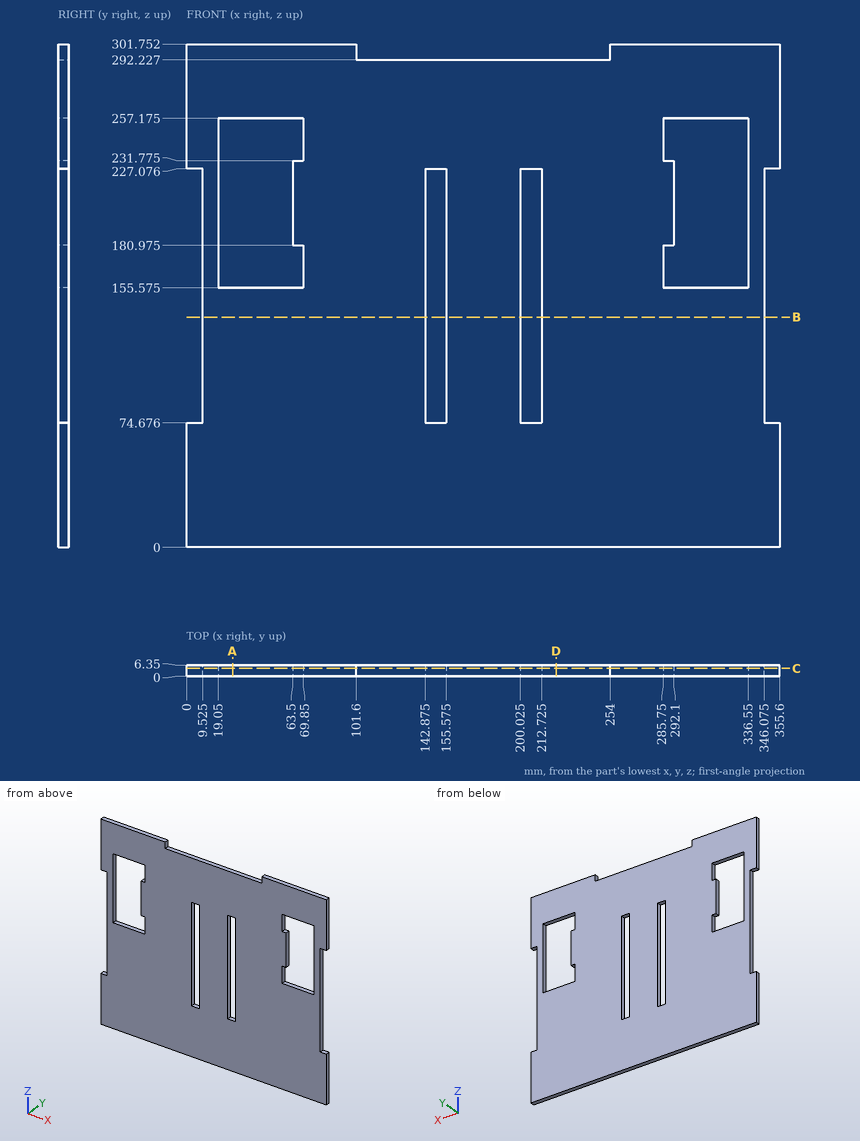
For this review, use the dimensioned drawing (mm, ordinates from the lowest corner) and the shaded views. Give positions to 0.01 mm unless a question says otherwise; leave off trailing zeros. Write each loop counter-clockwise with the first axis right and the second up, starting at its lowest first coordinate (ties: lowest second). Pieces come first, ordered by that corner, then holes. Notation, with made-up numbers: M -11,55.25 L 15,55.25 A33 cw 15,91.25 Z; hole C 22,36.5 d9. An arc over 180 degrees is marked long. Answer as a JSON object with one key per item and string values. Group by question number.
Item 1: For probe 1 along X at (y, z) = (5.5, 159.5) (3 decimals); probe 2 along X at (y, z) = (1.25, 249); probe 3 along X at (y, z) = (3.75, 88) (3 decimals), list the stretches that pass through material, from the lowest coordinate up. Write a range as [from, to].
Item 2: Consider section C-C on y = 4.5. Count the separate pieces of the cut face and the enclosed holes in it, plus the area to 3 significant figures.
Item 3: Consider section A-A on x = 27.5. Write out the cut boundary in (y, z) (3 decimals).
Item 4: Consider section B-B on z = 138. Write out the cut boundary in (x, y) (3 decimals).
Item 5: For pin 1 Ø3 at (x, z) = (150.5, 225) entering from +Y; pin 2 Ø2 at (x, y) = (121.5, 2) entering from -Z; pin 3 Ø3 at (y, z) = (4, 158.5) entering from -X (3 decimals); pin 4 Ø1.9 at (x, y) = (203, 2.5) entering from +Z, all flat-tipped, find the tip position at first contact; note any pin that passes through.
Item 6: Consider section D-D on x = 221.5. Write out the cut boundary in (y, z), plus the area to 3 significant figures.
Check result:
{
 "1": {"probe 1": "x = [9.525, 19.05], [69.85, 142.875], [155.575, 200.025], [212.725, 285.75], [336.55, 346.075]", "probe 2": "x = [0, 19.05], [69.85, 285.75], [336.55, 355.6]", "probe 3": "x = [9.525, 142.875], [155.575, 200.025], [212.725, 346.075]"},
 "2": {"separate pieces": "1", "enclosed holes": "4", "area": "89,400 mm^2"},
 "3": {"outline": "M 0,0 L 6.35,0 L 6.35,155.575 L 0,155.575 Z; M 0,257.175 L 6.35,257.175 L 6.35,301.752 L 0,301.752 Z"},
 "4": {"outline": "M 9.525,0 L 142.875,0 L 142.875,6.35 L 9.525,6.35 Z; M 155.575,0 L 200.025,0 L 200.025,6.35 L 155.575,6.35 Z; M 212.725,0 L 346.075,0 L 346.075,6.35 L 212.725,6.35 Z"},
 "5": {"pin 1": "passes through", "pin 2": "stops at z = 0", "pin 3": "stops at x = 9.525", "pin 4": "stops at z = 292.23"},
 "6": {"outline": "M 0,0 L 6.35,0 L 6.35,292.23 L 0,292.23 Z", "area": "1,860 mm^2"}
}
